from build123d import *

# Parameters (mm, degrees)
F0_W     = 31.75
F0_H     = 80
F1_DEPTH = 31.75
F3_DEPTH = 31.751
F4_W     = 25.4
F4_H     = 10
F4_W_2   = 3.175
F4_H_2   = 43.2458060166
F5_DEPTH = 31.751
F6_W     = 47.7026679298
F6_H     = 12.140064659
F6_H_2   = 10.4135097936
F7_DEPTH = 31.751
F9_DEPTH = 31.751


with BuildPart() as f1:
    # F0 (on Top) → F1 (new body)
    with BuildSketch(Plane.XY):
        Rectangle(F0_W, F0_H)
    extrude(amount=F1_DEPTH)

    # F2 (on face) → F3 (cut, through all)
    with BuildSketch(Plane.YZ.offset(15.875)):
        with BuildLine():
            Line((20.065903716, 15.875), (25.065903716, 15.875))
            ThreePointArc((25.065903716, 15.875), (24.9899424811, 16.7432408883), (24.7643668199, 17.5851007166))
            Line((24.7643668199, 17.5851007166), (20.065903716, 15.875))
        make_face()
        with BuildLine():
            ThreePointArc((35, 20.2186558202), (31.479055467, 23.1730790793), (29.1809221376, 19.1925953903))
            ThreePointArc((29.1809221376, 19.1925953903), (32.520944533, 17.2642325612), (35, 20.2186558202))
        make_face()
        with BuildLine():
            ThreePointArc((24.7643668199, 17.5851007166), (15.141864951, 15.0067591117), (25.065903716, 15.875))
            Line((25.065903716, 15.875), (20.065903716, 15.875))
            Line((20.065903716, 15.875), (24.7643668199, 17.5851007166))
        make_face()
    extrude(amount=-F3_DEPTH, mode=Mode.SUBTRACT)

    # F4 (on face) → F5 (cut, through all)
    with BuildSketch(Plane.XY.offset(31.75)):
        with Locations((0, -45)):
            Rectangle(F4_W, F4_H)
        with Locations((14.2875, -18.3770969917)):
            Rectangle(F4_W_2, F4_H_2)
        with Locations((-14.2875, -18.3770969917)):
            Rectangle(F4_W_2, F4_H_2)
    extrude(amount=-F5_DEPTH, mode=Mode.SUBTRACT)

    # F6 (on face) → F7 (cut, through all)
    with BuildSketch(Plane.YZ.offset(15.875)):
        with Locations((-20.6055279483, 34.6450323295)):
            Rectangle(F6_W, F6_H)
        with Locations((-20.6055279483, -2.0317548968)):
            Rectangle(F6_W, F6_H_2)
    extrude(amount=-F7_DEPTH, mode=Mode.SUBTRACT)

    # F8 (on face) → F9 (cut, through all)
    with BuildSketch(Plane.XY.offset(31.75)):
        Polygon((15.875, 3.2458060166), (15.875, 40), (7.125, 40), (7.125, 11.9958060166), align=None)
    extrude(amount=-F9_DEPTH, mode=Mode.SUBTRACT)


solid = f1.part
Verification items for the finished model (mm, model axes). A direction names the side the tool comes from. Give positions to 0.01 mm unless a question says otherwise; leave off trailing zeros. Loops run counter-clockwise (first coordinate to the right, second up) from the corner with the lowest first, then second, coordinate; pieces in that order, holes last. Notation, with made-up numbers: (-4, -25.5) - (25, -25.5) arc R21 cw to (25, 10.5) - close; hole circle Ø2 at (-4.5, 1). An arc over 180 degrees is marked (long way). Write item = value, one per line. Start each with the question number.
Q1. Tool access check on faces 4 (the face through (-12.7, -19, 16)), 5 (the face through (7.125, 26, 16)), 6 (the face through (12.7, -19, 16)), 7 (the face through (0, -19, 28.575)), 8 (the face through (0, -19, 3.175)). Record the directions out of +Z, -Z, +X, -X, +Y, -Y that give a thin tool (end or side, any length) a straight path to the whole face; none if there is none.
Q2. Thickness scan on line 1 (Z direction, x = -9, y = 32); line 2 (Y direction, x = -12, z = 20.5); line 3 (X direction, y = -36, z = 16.5). Record the ranges inside material, lowest first.
Q3. Cross-section at A-A, the plane y = 32. Enter the section's corners in (x, z) (3 decimals).
Q4. Depth check by flat-ended pin: P1, Ø16, axis at y = 20.07, z = 15.87, coming from the +X side (3 decimals); P2, Ø12, axis at y = 11, z = 13, coming from the +X side; P3, Ø12, axis at x = -8.5, y = -31.5, coming from the +Z side (3 decimals). Enter the tip coordinate at first touch or a pass-through.
Q5. Cross-section at D-D, the plane z = 12. Enter the section's corners in (x, y) (3 decimals), and give its area (3 significant figures).
Q6. Cross-section at B-B, the plane x = -8.5. Enter the section's corners in (y, z) (3 decimals), and give its area (3 significant figures).
Q7. Mould release check, pull along Y, two halves, no side actions. Record for faces 1 (the face through (0, -40, 16)), 2 (the face through (-4, 22, 31.75)), 3 (the face through (11.44, 7.68, 16.1)): released by +Y, released by -Y, zero draft, split by the parting line, or undercut.
Q8. Cross-section at C-C, the plane z = 8.5. Enter the section's corners in (x, y) (3 decimals).
Answer key:
q1.face_4 = +Z, -Z, -X, -Y
q1.face_5 = +Z, -Z, +X, +Y
q1.face_6 = +Z, -Z, +X, -Y
q1.face_7 = +Z, +X, -X, -Y
q1.face_8 = -Z, +X, -X, -Y
q2.line_1 = 0 to 17.22, 23.22 to 31.75
q2.line_2 = -40 to 18.17, 21.97 to 29.01, 34.99 to 40
q2.line_3 = -12.7 to 12.7
q3.outline = (-15.875, 0) - (7.125, 0) - (7.125, 17.219) - (-15.875, 17.219) - close; (-15.875, 23.219) - (7.125, 23.219) - (7.125, 31.75) - (-15.875, 31.75) - close
q4.P1 = 7.125
q4.P2 = 14.12
q4.P3 = 28.575
q5.outline = (-15.875, 3.246) - (-12.7, 3.246) - (-12.7, -40) - (12.7, -40) - (12.7, 3.246) - (15.875, 3.246) - (7.125, 11.996) - (7.125, 16.906) - (-15.875, 16.906) - close; (-15.875, 23.226) - (7.125, 23.226) - (7.125, 40) - (-15.875, 40) - close
q5.area = 1,840 mm^2
q6.outline = (-40, 3.175) - (3.246, 3.175) - (3.246, 0) - (40, 0) - (40, 31.75) - (3.246, 31.75) - (3.246, 28.575) - (-40, 28.575) - close; hole circle Ø10 at (20.066, 15.875); hole circle Ø6 at (32, 20.219)
q6.area = 2,160 mm^2
q7.face_1 = released by -Y
q7.face_2 = zero draft
q7.face_3 = released by +Y
q8.outline = (-15.875, 3.246) - (-12.7, 3.246) - (-12.7, -40) - (12.7, -40) - (12.7, 3.246) - (15.875, 3.246) - (7.125, 11.996) - (7.125, 40) - (-15.875, 40) - close
